Check sheet for the modelled part. Datum: model origin and axes. Units: mm. A direction names the side the tool comes from. Coordinates: 2 decimals unless noted, no trailing zeros. Order: outer loops, then holes, each group sorted by start corner. A loop starts at its lowest first (then second) coordinate and runs counter-clockwise, first axis right, second up. Notation, with made-up numbers: M 71.25,-27.75 L 110.25,-27.75 A29 cw 110.25,5.25 Z; hole C -31,15.25 d10. An arc over 180 degrees is marked long. Answer in a Markdown table with one row per item. Add a question column.
from build123d import *

# Parameters (mm, degrees)
SKETCH2_R   = 15
FRAME_DEPTH = 8


with BuildPart() as part:
    # Sketch2 → frame (new body)
    with BuildSketch(Plane(origin=(0, 0, 0), x_dir=(0, 0, -1), z_dir=(1, 0, 0))):
        with BuildLine():
            Line((0, -34), (-123, -23.238894386))
            Line((-123, -23.238894386), (-123, 148))
            Line((-123, 148), (92, 148))
            Line((92, 148), (92, 42))
            ThreePointArc((92, 42), (92.902828006, 40.076710729), (94.959233297, 39.542540991))
            ThreePointArc((94.959233297, 39.542540991), (102.025285395, 34.301898835), (96.270058953, 27.648268918))
            Line((96.270058953, 27.648268918), (85.887505091, 27.286969807))
            ThreePointArc((85.887505091, 27.286969807), (82.464905993, 25.763505578), (81.06139321, 22.289994429))
            Line((81.06139321, 22.289994429), (81.06139321, -1.710005571))
            ThreePointArc((81.06139321, -1.710005571), (82.112283863, -4.412366401), (84.712770239, -5.694784363))
            Line((84.712770239, -5.694784363), (96.584327666, -6.733411056))
            ThreePointArc((96.584327666, -6.733411056), (102.057738172, -12.501182265), (97, -18.636709289))
            Line((97, -18.636709289), (0, -34))
        make_face()
        Circle(SKETCH2_R, mode=Mode.SUBTRACT)
        with BuildLine():
            Line((-113, -3.558496414), (-113, 45.220981939))
            ThreePointArc((-113, 45.220981939), (-110.113091309, 49.752520874), (-104.786061952, 49.051204155))
            Line((-104.786061952, 49.051204155), (-38.667003468, -6.429273433))
            ThreePointArc((-38.667003468, -6.429273433), (-37.261543853, -12.172912811), (-42.31672023, -15.240469139))
            Line((-42.31672023, -15.240469139), (-107.522934456, -9.535664603))
            ThreePointArc((-107.522934456, -9.535664603), (-111.423664021, -7.61203766), (-113, -3.558496414))
        make_face(mode=Mode.SUBTRACT)
        with BuildLine():
            Line((-113, 71.795435384), (-113, 121.054164621))
            ThreePointArc((-113, 121.054164621), (-109.586523282, 125.795782897), (-104.00682245, 124.063239737))
            Line((-104.00682245, 124.063239737), (-33.611864664, 30.645975539))
            ThreePointArc((-33.611864664, 30.645975539), (-34.821190136, 16.092200216), (-49.418311221, 15.646217831))
            Line((-49.418311221, 15.646217831), (-110.856725658, 67.199168725))
            ThreePointArc((-110.856725658, 67.199168725), (-112.437846722, 69.259725813), (-113, 71.795435384))
        make_face(mode=Mode.SUBTRACT)
        with BuildLine():
            Line((-91.959119468, 138), (52.842661319, 138))
            ThreePointArc((52.842661319, 138), (57.105862141, 135.612492824), (57.29769394, 130.730047501))
            Line((57.29769394, 130.730047501), (17.87282228, 53.354380202))
            ThreePointArc((17.87282228, 53.354380202), (-7.155112396, 36.472825104), (-34.734267785, 48.7518562))
            Line((-34.734267785, 48.7518562), (-95.952297019, 129.990924884))
            ThreePointArc((-95.952297019, 129.990924884), (-96.433791276, 135.230989066), (-91.959119468, 138))
        make_face(mode=Mode.SUBTRACT)
        with BuildLine():
            Line((66.06139321, 100.911084489), (66.06139321, 47.537774319))
            ThreePointArc((66.06139321, 47.537774319), (65.149681787, 44.358258734), (62.69162009, 42.145010042))
            Line((62.69162009, 42.145010042), (30.109631358, 26.253712336))
            ThreePointArc((30.109631358, 26.253712336), (21.653823385, 27.706685885), (20.348645329, 36.186563882))
            Line((20.348645329, 36.186563882), (54.715354065, 103.635027487))
            ThreePointArc((54.715354065, 103.635027487), (61.462065393, 106.745304011), (66.06139321, 100.911084489))
        make_face(mode=Mode.SUBTRACT)
        with BuildLine():
            Line((66.06139321, 23.060531629), (66.06139321, -2.212977084))
            ThreePointArc((66.06139321, -2.212977084), (64.623829003, -6.109665374), (61, -8.139107128))
            Line((61, -8.139107128), (49.27069142, -9.996847102))
            ThreePointArc((49.27069142, -9.996847102), (31.689538707, 0.882700312), (39.850923857, 19.878838738))
            Line((39.850923857, 19.878838738), (57.431166329, 28.453295907))
            ThreePointArc((57.431166329, 28.453295907), (63.240908795, 28.148820206), (66.06139321, 23.060531629))
        make_face(mode=Mode.SUBTRACT)
    extrude(amount=FRAME_DEPTH)


solid = part.part
1. Section check A-A on x = 4. State how many separate pieces and enclosed holes the cut face has, then the cut area to 3 significant figures.
2. Set-up check for faces 1 (the flat face through (3.944, -6.207, -90.565)), 2 (the flat face through (3.94, -26.21, -49.18)), 3 (the cylindrical face through (3.94, 135.16, 96.47)): record each of +Z, -Z, +X, -X, +Y, -Y from which the full face is reachable in a straight line by a thin tool's end or side.
3. Section check B-B on z = -71. Enter the section's corners in (x, y).
4. Go/stop test with flat-tipped pins: pin 1 Ø2 at (x, y) = (6.5, 90) entering from -Z; pin 2 Ø2 at (x, z) = (3, 49) entering from -Y; pin 3 Ø4 at (x, z) = (5, 36) entering from -Y. Record where each tip stops, or that it passes through.
5. Release check for a two-part mould opening along Y. For faces 4 (the cylindrical face through (3.9, 25.8, -82.5)), 5 (the flat face through (4, 148, 17)), 6 (the flat face through (8, 38, -16)), 7 (the flat face through (4, 96, 113)) record: released by +Y, released by -Y, zero draft, split by the parting line, or undercut.
6. Scan lines: line 1 (Z direction, x = 0.75, y = 15.5); line 2 (Y direction, x = 4.75, z = 74); line 3 (Y direction, x = 3.25, z = 0). Record each from-to range of solid material in increasing order.
Result sheet:
| question | item | result |
|---|---|---|
| 1 | separate pieces | 1 |
| 1 | enclosed holes | 6 |
| 1 | area | 17,500 mm^2 |
| 2 | face 1 | -Z, +X, -X |
| 2 | face 2 | -Z, +X, -X, -Y |
| 2 | face 3 | +X, -X |
| 3 | outline | M 0,-22.75 L 8,-22.75 L 8,148 L 0,148 Z |
| 4 | pin 1 | z = -92 |
| 4 | pin 2 | y = -29.8 |
| 4 | pin 3 | y = -31.03 |
| 5 | face 4 | undercut |
| 5 | face 5 | released by +Y |
| 5 | face 6 | zero draft |
| 5 | face 7 | undercut |
| 6 | line 1 | -81.06 to -66.06, -34.4 to 35.5, 49.24 to 64.8, 113 to 123 |
| 6 | line 2 | -27.53 to -12.47, 23.22 to 36.27, 84.24 to 100.86, 138 to 148 |
| 6 | line 3 | -34 to -15, 15 to 37.96, 138 to 148 |
